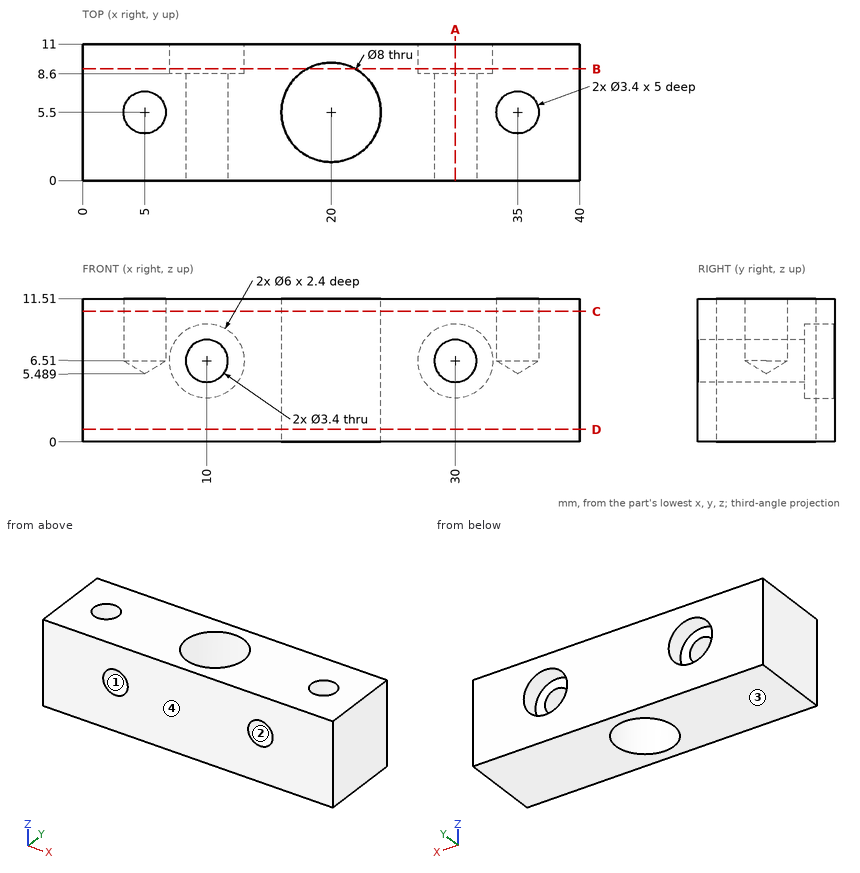
Input: dimensioned drawing with shaded views. Units: mm. Origin: part minimum x, y, z. Coordinates: 2 decimals unless noted, no trailing zeros. Order: outer loops, then holes, each group sorted by start corner. A loop starts at its lowest first (then second) coordinate and runs counter-clockwise, first axis right, second up. Notation, with made-up numbers: (13, 50) - (39, 50) arc R24 ccw to (39, 65) - close; hole circle Ø11 at (89.25, -1.5). An arc over 180 degrees is marked (long way). One line per item, written item: value.
1) Cut plane A-A on x = 30. Output: boundary loops of the cut face in (y, z).
Computed values:
outline: (0, 0) - (11, 0) - (11, 3.51) - (8.6, 3.51) - (8.6, 4.81) - (0, 4.81) - close; (0, 8.21) - (8.6, 8.21) - (8.6, 9.51) - (11, 9.51) - (11, 11.51) - (0, 11.51) - close
2) Contact query for flat-ended pins moving along their axis: pin 1 (5 mm diameter, centred on x = 10, z = 6.51, fed in from +Y); pin 2 (3 mm diameter, centred on x = 10, z = 6.51, fed in from -Y); pin 3 (2.5 mm diameter, centred on x = 5, y = 5.5, fed in from +Z); pin 4 (3 mm diameter, centred on x = 35, y = 5.5, fed in from +Z). Output: stop coordinate, or through.
Computed values:
pin 1: stops at y = 8.6
pin 2: passes through
pin 3: stops at z = 6.24
pin 4: stops at z = 6.39
3) Mould query, pull axis Z, two halves, no side actions, for the marked faces 1, 2, 3 and 4. Classes: released by +Z, released by -Z, zero draft, split by the parting line, or undercut.
Computed values:
face 1: undercut
face 2: undercut
face 3: released by -Z
face 4: zero draft
4) Cut plane C-C on z = 10.5. Output: boundary loops of the cut face in (x, y).
Computed values:
outline: (0, 0) - (40, 0) - (40, 11) - (0, 11) - close; hole circle Ø3.4 at (5, 5.5); hole circle Ø8 at (20, 5.5); hole circle Ø3.4 at (35, 5.5)
5) Ray query, line 1 (X direction, y = 5.5, z = 9.55); line 2 (X direction, y = 8.25, z = 6.5) (1 decimal); line 3 (Y direction, x = 35, z = 10.35). Return the intervals inside material, ascending. Write a range as [from, to].
Computed values:
line 1: x = [0, 3.3], [6.7, 16], [24, 33.3], [36.7, 40]
line 2: x = [0, 8.3], [11.7, 17.1], [22.9, 28.3], [31.7, 40]
line 3: y = [0, 3.8], [7.2, 11]
6) Cut plane D-D on z = 1. Output: boundary loops of the cut face in (x, y).
Computed values:
outline: (0, 0) - (40, 0) - (40, 11) - (0, 11) - close; hole circle Ø8 at (20, 5.5)
7) Cut plane B-B on y = 9. Output: boundary loops of the cut face in (x, z), plus the area to 3 significant figures.
Computed values:
outline: (0, 0) - (18.06, 0) - (18.06, 11.51) - (0, 11.51) - close; (21.94, 0) - (40, 0) - (40, 11.51) - (21.94, 11.51) - close; hole circle Ø6 at (10, 6.51); hole circle Ø6 at (30, 6.51)
area: 359 mm^2
